from build123d import *

# Parameters (mm, degrees)
F1_DEPTH = 5
F2_DEPTH = 2
F3_DEPTH = 2
F4_D     = 2
F5_R     = 1


with BuildPart() as f1:
    # F0 (on Top) → F1 (new body)
    with BuildSketch(Plane.XY):
        with BuildLine():
            ThreePointArc((4.582576, 2), (-4.894532, -1.021548), (5, 0))
            ThreePointArc((5, 0), (4.894532, 1.021548), (4.582576, 2))
        make_face()
    extrude(amount=F1_DEPTH)

    # F0 (on Top) → F2 (join)
    with BuildSketch(Plane.XY):
        with BuildLine():
            ThreePointArc((4.582576, 2), (4.894532, 1.021548), (5, 0))
            Line((5, 0), (9.582576, 0))
            Line((9.582576, 0), (9.582576, 2))
            Line((9.582576, 2), (4.582576, 2))
        make_face()
    extrude(amount=F2_DEPTH)

    # F0 (on Top) → F3 (join, symmetric)
    with BuildSketch(Plane.XY):
        Polygon((9.582576, 2), (9.582576, 0), (14.778728, 0), (14.778728, 1), (9.582576, 4), align=None)
    extrude(amount=F3_DEPTH, both=True)

    # F4 (through all)
    with Locations(Plane(origin=(0, 0, 0), x_dir=(1, 0, 0), z_dir=(0, 0, -1))):
        with Locations((0, 0)):
            Hole(F4_D / 2)

    # F5
    f5_edges = [f1.edges().sort_by_distance(p)[0] for p in [
        (9.582576, 4, 0),
    ]]
    fillet(f5_edges, radius=F5_R)


solid = f1.part
For this review, take the finished solid that the model builds, in its own axes (mm). A direction names the side the tool comes from. Round coordinates to 2 decimals unless told otherwise and drop trailing zeros. Order: outer loops, then holes, each group sorted by start corner. A loop starts at its lowest first (then second) coordinate and runs counter-clockwise, first axis right, second up. Notation, with made-up numbers: M 40.25,0 L 84.25,0 A16 cw 84.25,12 Z; hole C 47,44 d6. An arc over 180 degrees is marked long. Write each question's results on one line, items separated by ' | '. Start each with the question number.
1. Clearance check with flat-ended pins moving along their axes: pin 1 Ø3 at (y, z) = (3, 1) entering from +X; pin 2 Ø0.7 at (y, z) = (1.5, 0.5) entering from -X; pin 3 Ø1.6 at (x, z) = (6, 1) entering from +Y; pin 4 Ø5 at (x, y) = (12, -3.5) entering from -Z. State where each tip first meets the part, or that it passes through.
2. Add section D-D (x = 3). State the section outline as (y, z) points.
3. Tool access review of faces 1 (the face through (9.583, 1, -1)), 2 (the face through (4.9, 1, 3.5)), 3 (the face through (11, 0, 0)), 4 (the face through (-0.1, 1.2, 5)): name each direction out of +Z, -Z, +X, -X, +Y, -Y from which nothing blocks a thin tool from reaching the whole face with its end or side.
4. Add section B-B (z = 1.5). State the section outline as (x, y) points.
5. Add section A-A (x = 0). State the section outline as (y, z) points.
6. Add section C-C (y = 0.75). State the section outline as (x, z) points, then the cut area to 3 significant figures.
7. To check wall thickness, follow L1, parallel to Y at x = 0, z = 3.65; L2, parallel to Z at x = -1, y = -4; L3, parallel to X at y = 0.5, z = -1. State the ranges of each line that lie inside material, in increasing order. Write a range as [from, to].
8. Draft analysis for pull direction X (two halves, no side actions). For faces 5 (the face through (1, -1, 0)), 6 (the face through (7, 2, 1)), 7 (the face through (12.96, 2.05, 0.03)), state which applies: pulls with the +X half, pulls with the -X half, needs draft (parallel to the pull), parting line crosses it, or undercut.
Output values:
1) pin 1: x = 13.91 | pin 2: x = -4.87 | pin 3: y = 2 | pin 4: through
2) outline: M -4,0 L 4,0 L 4,5 L -4,5 Z
3) face 1: -Z, +Y | face 2: +Z, +X, +Y | face 3: +Z, -Z, +X, -Y | face 4: +Z, +X, -X, +Y, -Y
4) outline: M 4.58,2 A5 ccw long 5,0 L 14.78,0 L 14.78,1 L 11.08,3.13 A1 ccw 9.58,2.27 L 9.58,2 Z; hole C 0,0 d2
5) outline: M -5,0 L -1,0 L -1,5 L -5,5 Z; M 1,0 L 5,0 L 5,5 L 1,5 Z
6) outline: M -4.94,0 L -0.66,0 L -0.66,5 L -4.94,5 Z; M 0.66,0 L 9.58,0 L 9.58,-2 L 14.78,-2 L 14.78,2 L 4.94,2 L 4.94,5 L 0.66,5 Z | area: 72.9 mm^2
7) L1: [-5, -1], [1, 5] | L2: [0, 5] | L3: [9.58, 14.78]
8) face 5: needs draft | face 6: undercut | face 7: pulls with the +X half
